Read the model definition and answer for the solid it produces. Units are mm, in the model's axes. Give positions to 0.01 mm unless a question says otherwise; leave off trailing zeros. Write each loop counter-clockwise with the first axis right and the second up, starting at its lowest first coordinate (ties: lowest second). Pieces come first, ordered by that corner, then holes. Notation, with made-up numbers: (37, -7.5) - (65, -7.5) arc R23 ccw to (65, 28.5) - close; hole circle Ø4 at (-17, -13). An arc over 180 degrees is marked (long way). Answer as CSV lines item,"result".
```python
from build123d import *

# Parameters (mm, degrees)
BOSS_EXTRUDE1_DEPTH = 10
BOSS_EXTRUDE1_TAPER = 8


with BuildPart() as part:
    # Sketch1 → Boss-Extrude1 (new body)
    with BuildSketch(Plane.XY):
        with BuildLine():
            ThreePointArc((-6.897446528, 3.888888889), (-8.305608926, 3.305608926), (-8.888888889, 1.897446528))
            Line((-8.888888889, 1.897446528), (-8.888888889, -4.11966875))
            ThreePointArc((-8.888888889, -4.11966875), (-8.305608926, -5.527831148), (-6.897446528, -6.111111111))
            Line((-6.897446528, -6.111111111), (-0.88033125, -6.111111111))
            ThreePointArc((-0.88033125, -6.111111111), (0.527831148, -5.527831148), (1.111111111, -4.11966875))
            Line((1.111111111, -4.11966875), (1.111111111, 1.897446528))
            ThreePointArc((1.111111111, 1.897446528), (0.527831148, 3.305608926), (-0.88033125, 3.888888889))
            Line((-0.88033125, 3.888888889), (-6.897446528, 3.888888889))
        make_face()
    extrude(amount=BOSS_EXTRUDE1_DEPTH, taper=BOSS_EXTRUDE1_TAPER)


solid = part.part
```
(1) A cutting plane is placed at B-B (x = -2). Write down the section's boundary in (y, z), and give its area (3 significant figures).
Worked out:
outline,"(-6.11, 0) - (3.89, 0) - (2.48, 10) - (-4.71, 10) - close"
area,"85.9 mm^2"
(2) Find the intervals of material crossed by L1, parallel to Y at x = -1.25, z = 5.5; L2, parallel to Y at x = -7, z = 9.5; L3, parallel to X at y = 0, z = 1, in increasing order.
Worked out:
L1,"y = -5.34 to 3.12"
L2,"y = -4.77 to 2.55"
L3,"x = -8.75 to 0.97"
(3) A cutting plane is placed at D-D (z = 4). Write down the section's boundary in (x, y).
Worked out:
outline,"(-8.33, -4.12) arc R1.43 ccw to (-6.9, -5.55) - (-0.88, -5.55) arc R1.43 ccw to (0.55, -4.12) - (0.55, 1.9) arc R1.43 ccw to (-0.88, 3.33) - (-6.9, 3.33) arc R1.43 ccw to (-8.33, 1.9) - close"
(4) A cutting plane is placed at C-C (y = 1.25). Write down the section's boundary in (x, z), and give its area (3 significant figures).
Worked out:
outline,"(-8.89, 0) - (1.11, 0) - (-0.29, 10) - (-7.48, 10) - close"
area,"85.9 mm^2"
(5) A cutting plane is placed at A-A (z = 9). Write down the section's boundary in (x, y), and give its area (3 significant figures).
Worked out:
outline,"(-7.62, -4.12) arc R0.73 ccw to (-6.9, -4.85) - (-0.88, -4.85) arc R0.73 ccw to (-0.15, -4.12) - (-0.15, 1.9) arc R0.73 ccw to (-0.88, 2.62) - (-6.9, 2.62) arc R0.73 ccw to (-7.62, 1.9) - close"
area,"55.4 mm^2"
(6) Each of these flat-tipped pins is pushed along its axis until it touches: P1, Ø4, axis at x = -6, z = 2.5, coming from the +Y side; P2, Ø4, axis at y = -1, z = 3.5, coming from the +X side; P3, Ø1.5, axis at x = -1.5, z = 7, coming from the +Y side; P4, Ø5, axis at x = -6.5, z = 1.5, coming from the -Y side. Where does it stop, or does it pass through?
Worked out:
P1,"stops at y = 3.82"
P2,"stops at x = 0.9"
P3,"stops at y = 3.01"
P4,"stops at y = -6.11"
